For this review, take the finished solid that the model builds, in its own axes (mm). Coordinates: 2 decimals unless noted, no trailing zeros. Loops run counter-clockwise (first coordinate to the right, second up) from the corner with the lowest first, then second, coordinate; pieces in that order, holes last. Notation, with made-up numbers: (-11, -36) - (-3, -36) arc R10 cw to (-3, -27) - close; hole circle Ø2 at (45.5, 87.5). An arc over 180 degrees is marked (long way). One line per item, written item: value. Start each with the question number.
1. Take a section at C-C, the plane z = 916. State the section outline as (x, y) points, and give its area (3 significant figures).
2. Take a section at B-B, the plane x = 861. State the section outline as (y, z) points.
3. To check wall thickness, follow line 1 (Y direction, x = 762, z = 916.75); line 2 (X direction, y = 1147.5, z = 917); line 3 (Y direction, x = 968, z = 919.25). State the ranges of each line that lie inside material, in increasing order. Write a range as from..to.
4. Take a section at A-A, the plane y = 1150. State the section outline as (x, z) points, and give its area (3 significant figures).
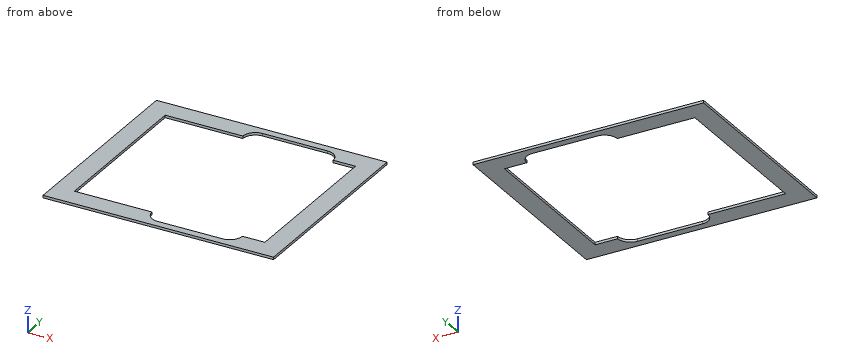
```python
from build123d import *

# Parameters (mm, degrees)
SKETCH_W  = 584.2
SKETCH_H  = 508
PAD_DEPTH = 6.35


with BuildPart() as part:
    # Sketch → Pad (new body)
    with BuildSketch(Plane(origin=(914.4, 1066.8, 914.4), x_dir=(1, 0, 0), z_dir=(0, 0, 1))):
        Rectangle(SKETCH_W, SKETCH_H)
        with BuildLine():
            Line((241.3, -203.2), (241.3, 203.2))
            Line((241.3, 203.2), (184.15, 203.2))
            ThreePointArc((184.15, 203.2), (174.85064, 225.65064), (152.4, 234.95))
            Line((-12.7, 234.95), (152.4, 234.95))
            ThreePointArc((-12.7, 234.95), (-35.15064, 225.65064), (-44.45, 203.2))
            Line((-241.3, 203.2), (-44.45, 203.2))
            Line((-241.3, 203.2), (-241.3, -203.2))
            Line((-241.3, -203.2), (-44.45, -203.2))
            ThreePointArc((-44.45, -203.2), (-35.15064, -225.65064), (-12.7, -234.95))
            Line((-12.7, -234.95), (152.4, -234.95))
            ThreePointArc((152.4, -234.95), (174.85064, -225.65064), (184.15, -203.2))
            Line((241.3, -203.2), (184.15, -203.2))
        make_face(mode=Mode.SUBTRACT)
    extrude(amount=PAD_DEPTH)


solid = part.part
```
Solutions:
1. outline: (622.3, 812.8) - (1206.5, 812.8) - (1206.5, 1320.8) - (622.3, 1320.8) - close; hole (673.1, 863.6) - (869.95, 863.6) arc R31.75 ccw to (901.7, 831.85) - (1066.8, 831.85) arc R31.75 ccw to (1098.55, 863.6) - (1155.7, 863.6) - (1155.7, 1270) - (1098.55, 1270) arc R31.75 ccw to (1066.8, 1301.75) - (901.7, 1301.75) arc R31.75 ccw to (869.95, 1270) - (673.1, 1270) - close
1. area: 87,000 mm2
2. outline: (812.8, 914.4) - (863.6, 914.4) - (863.6, 920.75) - (812.8, 920.75) - close; (1270, 914.4) - (1320.8, 914.4) - (1320.8, 920.75) - (1270, 920.75) - close
3. line 1: 812.8..863.6, 1270..1320.8
3. line 2: 622.3..673.1, 1155.7..1206.5
3. line 3: 812.8..831.85, 1301.75..1320.8
4. outline: (622.3, 914.4) - (673.1, 914.4) - (673.1, 920.75) - (622.3, 920.75) - close; (1155.7, 914.4) - (1206.5, 914.4) - (1206.5, 920.75) - (1155.7, 920.75) - close
4. area: 645 mm2
